Geometry: final body of the model. Coordinates: model frame, mm. A direction names the side the tool comes from. Give positions to 0.01 mm unless a question says otherwise; leave off trailing zeros. Loops run counter-clockwise (first coordinate to the right, second up) from the corner with the lowest first, then second, coordinate; pieces in that order, holes last. Notation, with made-up numbers: (2, 55) -> (59, 55) arc R19 ccw to (59, 65) -> close; hole circle Ø3 at (61, 21.25). An arc over 180 degrees is marked (long way). Answer in a Markdown table with one row per item. Add a question column.
1) Section query D-D (x = 2.5). Return the cut outline in (y, z), plus the area to 3 significant figures.
2) First-contact query: P1, Ø6.5, axis at x = 17.5, z = 2.5, coming from the +Y side; P2, Ø12.5, axis at x = 20, y = -4.5, coming from the +Z side; P3, Ø3, axis at x = 20, y = -7.5, coming from the -Z side; P4, Ø1.8, axis at y = -14, z = -33.97, coming from the +X side. Flat tips, straight axial feed; report the tip coordinate or a pass-through.
3) Section query A-A (x = 14.25). Return the cut outline in (y, z).
4) Section query C-C (y = -1.75). Return the cut outline in (x, z).
5) Draft query along Z for faces 5 (the flat face through (5, 8.298, 3)), 6 (the flat face through (5.423, -13.385, -37.984)), 7 (the flat face through (11, -3, 3)). Return one class per face: +Z half, -Z half, draft (parallel to the pull), parting line (faces both ways), or undercut.
6) Access query for faces 1 (the flat face through (17, 4.548, 3)), 2 (the cylindrical face through (17.59, 4.45, -6.93)), 3 (the cylindrical face through (17.591, -10.882, 13.394)), 4 (the flat face through (17, -3, 13.996)). Directions: +Z, -Z, +X, -X, +Y, -Y. A direction counts if a zero-diameter tool reaches every point of the face in a straight line with its end or side. Return the directions, or none.
7) Line query: line 1 (Y direction, x = 22.25, z = -1); line 2 (Z direction, x = 18.5, y = 1.5); line 3 (X direction, y = -1.25, z = -11.5). Output: solid intervals per line, ascending. Write a range as from..to.
8) Section query B-B (z = -3.5). Return the cut outline in (x, y).
```python
from build123d import *

# Parameters (mm, degrees)
SKETCH1_R           = 1
BOSS_EXTRUDE1_DEPTH = 11
SKETCH2_W           = 21.5
SKETCH2_H           = 16.5
SKETCH2_W_2         = 20.5
SKETCH2_H_2         = 15.5
EXTRUDE_THIN1_DEPTH = 13
FILLET1_R           = 2
FILLET2_R           = 2


with BuildPart() as part:
    # Sketch1 → Boss-Extrude1 (new body)
    with BuildSketch(Plane(origin=(0, 0, 0), x_dir=(0, 0, -1), z_dir=(1, 0, 0))):
        Polygon((-21.745526202, 8.298037657), (-48.335335533, 3.60953686), (-48.335335533, -8.949767561), (-40.456873509, -18.001277719), (-21.745526202, -14.701962343), (15.254473798, -14.701962343), (33.965821106, -18.001277719), (41.84428313, -8.949767561), (41.84428313, 3.60953686), (15.254473798, 8.298037657), align=None)
        with Locations((-40.456873509, -14.001277719)):
            Circle(SKETCH1_R, mode=Mode.SUBTRACT)
        with Locations((33.965821106, -14.001277719)):
            Circle(SKETCH1_R, mode=Mode.SUBTRACT)
    extrude(amount=BOSS_EXTRUDE1_DEPTH)

    # Sketch2 → Extrude-Thin1 (add)
    with BuildSketch(Plane(origin=(11, 0, 0), x_dir=(0, 0, -1), z_dir=(1, 0, 0))):
        with Locations((-3.245526202, -3.201962343)):
            Rectangle(SKETCH2_W, SKETCH2_H)
        with Locations((-3.245526202, -3.201962343)):
            Rectangle(SKETCH2_W_2, SKETCH2_H_2, mode=Mode.SUBTRACT)
    extrude(amount=EXTRUDE_THIN1_DEPTH)

    # Fillet1
    fillet1_edges = [part.edges().sort_by_distance(p)[0] for p in [
        (5.5, 8.298037657, -15.254473798),
        (5.5, 3.60953686, -41.84428313),
        (5.5, -8.949767561, -41.84428313),
        (5.5, -18.001277719, -33.965821106),
        (5.5, -14.701962343, -15.254473798),
        (5.5, -14.701962343, 21.745526202),
        (5.5, -18.001277719, 40.456873509),
        (5.5, -8.949767561, 48.335335533),
        (5.5, 3.60953686, 48.335335533),
        (5.5, 8.298037657, 21.745526202),
    ]]
    fillet(fillet1_edges, radius=FILLET1_R)

    # Fillet2
    fillet2_edges = [part.edges().sort_by_distance(p)[0] for p in [
        (17.5, -11.451962343, -7.504473798),
        (17.5, 5.048037657, -7.504473798),
        (17.5, 5.048037657, 13.995526202),
        (17.5, -11.451962343, 13.995526202),
        (17.5, 4.548037657, -7.004473798),
        (17.5, 4.548037657, 13.495526202),
        (17.5, -10.951962343, 13.495526202),
        (17.5, -10.951962343, -7.004473798),
    ]]
    fillet(fillet2_edges, radius=FILLET2_R)


solid = part.part
```
Evaluation:
| question | item | result |
|---|---|---|
| 1 | outline | (-17.8, -32.85) arc R2 ccw to (-17.15, -34.71) -> (-9.51, -41.35) arc R2 ccw to (-8.2, -41.84) -> (1.93, -41.84) arc R2 ccw to (3.9, -40.19) -> (8.27, -15.43) arc R2 ccw to (8.3, -15.08) -> (8.3, 21.57) arc R2 ccw to (8.27, 21.92) -> (3.9, 46.68) arc R2 ccw to (1.93, 48.34) -> (-8.2, 48.34) arc R2 ccw to (-9.51, 47.84) -> (-17.15, 41.2) arc R2 ccw to (-17.8, 39.34) -> (-14.73, 21.92) arc R2 cw to (-14.7, 21.57) -> (-14.7, -15.08) arc R2 cw to (-14.73, -15.43) -> close; hole circle Ø2 at (-14, -33.97); hole circle Ø2 at (-14, 40.46) |
| 1 | area | 1,980 mm² |
| 2 | P1 | y = 5.05 |
| 2 | P2 | z = 14 |
| 2 | P3 | z = -7.5 |
| 2 | P4 | through |
| 3 | outline | (-11.45, -5.5) arc R2 ccw to (-9.45, -7.5) -> (3.05, -7.5) arc R2 ccw to (5.05, -5.5) -> (5.05, 12) arc R2 ccw to (3.05, 14) -> (-9.45, 14) arc R2 ccw to (-11.45, 12) -> close; hole (-10.95, -5) arc R2 ccw to (-8.95, -7) -> (2.55, -7) arc R2 ccw to (4.55, -5) -> (4.55, 11.5) arc R2 ccw to (2.55, 13.5) -> (-8.95, 13.5) arc R2 ccw to (-10.95, 11.5) -> close |
| 4 | outline | (0, -41.84) -> (11, -41.84) -> (11, -7.5) -> (24, -7.5) -> (24, -7) -> (11, -7) -> (11, 13.5) -> (24, 13.5) -> (24, 14) -> (11, 14) -> (11, 48.34) -> (0, 48.34) -> close |
| 5 | face 5 | draft |
| 5 | face 6 | -Z half |
| 5 | face 7 | undercut |
| 6 | face 1 | +X |
| 6 | face 2 | -Z, +X, +Y |
| 6 | face 3 | +Z, +X, -Y |
| 6 | face 4 | +Z, +X, +Y, -Y |
| 7 | line 1 | -11.45..-10.95, 4.55..5.05 |
| 7 | line 2 | -7.5..-7, 13.5..14 |
| 7 | line 3 | 0..11 |
| 8 | outline | (0, -14.7) -> (11, -14.7) -> (11, -11.45) -> (24, -11.45) -> (24, -10.95) -> (11, -10.95) -> (11, 4.55) -> (24, 4.55) -> (24, 5.05) -> (11, 5.05) -> (11, 8.3) -> (0, 8.3) -> close |
